```python
from build123d import *

# Parameters (mm, degrees)
SKETCH3_R                 = 2.5
BOSS_EXTRUDE1_DEPTH       = 62.34264779
CHAMFER1_SIZE             = 1.5
CHAMFER1_SIZE2            = 0.866025404
M3X0_5_TAPPED_HOLE1_D     = 2.5
M3X0_5_TAPPED_HOLE1_DEPTH = 4
M3X0_5_TAPPED_HOLE1_TIP   = 0.751075774
SKETCH7_R                 = 1.5
CUT_EXTRUDE1_DEPTH        = 3.5
CUT_EXTRUDE1_DEPTH_BACK   = 3.5
SKETCH8_W                 = 1
SKETCH8_H                 = 6
CUT_EXTRUDE2_DEPTH        = 3.5000001
CUT_EXTRUDE2_DEPTH_BACK   = 3.5000001
SKETCH9_R                 = 3
SKETCH9_R_2               = 2
CUT_EXTRUDE3_DEPTH        = 0.75


with BuildPart() as part:
    # Sketch3 → Boss-Extrude1 (new body)
    with BuildSketch(Plane(origin=(0, 0, 0), x_dir=(1, 0, 0), z_dir=(0, 1, 0))):
        Circle(SKETCH3_R)
    extrude(amount=BOSS_EXTRUDE1_DEPTH)

    # Chamfer1
    chamfer1_edges = [part.edges().sort_by_distance(p)[0] for p in [
        (-2.5, 62.34264779, 0),
    ]]
    chamfer1_side = [part.faces().sort_by_distance(p)[0] for p in [
        (-2.5, 31.171323895, 0),
    ]]
    chamfer(chamfer1_edges, length=CHAMFER1_SIZE, length2=CHAMFER1_SIZE2, reference=chamfer1_side[0])

    # M3x0.5 Tapped Hole1
    with Locations(Plane(origin=(0, 62.34264779, 0), x_dir=(1, 0, 0), z_dir=(0, 1, 0))):
        with Locations((0, 0)):
            Hole(M3X0_5_TAPPED_HOLE1_D / 2, depth=M3X0_5_TAPPED_HOLE1_DEPTH)
            with Locations((0, 0, -(M3X0_5_TAPPED_HOLE1_DEPTH + M3X0_5_TAPPED_HOLE1_TIP / 2))):  # 118° drill point
                Cone(0, M3X0_5_TAPPED_HOLE1_D / 2, M3X0_5_TAPPED_HOLE1_TIP, mode=Mode.SUBTRACT)

    # Sketch7 → Cut-Extrude1 (cut, two sides)
    with BuildSketch(Plane.XY) as cut_extrude1_sk:
        with Locations((0, 58.34264779)):
            Circle(SKETCH7_R)
    extrude(amount=CUT_EXTRUDE1_DEPTH, mode=Mode.SUBTRACT)
    extrude(cut_extrude1_sk.sketch, amount=-CUT_EXTRUDE1_DEPTH_BACK, mode=Mode.SUBTRACT)

    # Sketch8 → Cut-Extrude2 (cut, two sides)
    with BuildSketch(Plane.XY) as cut_extrude2_sk:
        with Locations((-2, 3)):
            Rectangle(SKETCH8_W, SKETCH8_H)
    extrude(amount=CUT_EXTRUDE2_DEPTH, mode=Mode.SUBTRACT)
    extrude(cut_extrude2_sk.sketch, amount=-CUT_EXTRUDE2_DEPTH_BACK, mode=Mode.SUBTRACT)

    # Sketch9 → Cut-Extrude3 (cut)
    with BuildSketch(Plane(origin=(0, 17.15, 0), x_dir=(1, 0, 0), z_dir=(0, 1, 0))):
        Circle(SKETCH9_R)
        Circle(SKETCH9_R_2, mode=Mode.SUBTRACT)
    extrude(amount=CUT_EXTRUDE3_DEPTH, mode=Mode.SUBTRACT)


solid = part.part
```
Can you work these out from the model? Positions are in its coordinate system, mm. A direction names the side the tool comes from. Give positions to 0.01 mm unless a question says otherwise; leave off trailing zeros. Loops run counter-clockwise (first coordinate to the right, second up) from the corner with the lowest first, then second, coordinate; pieces in that order, holes last. Notation, with made-up numbers: M -9.5,-38 L -2.5,-38 A23 cw -2.5,1 Z; hole C 85.25,-26.75 d7. An arc over 180 degrees is marked long. Answer in a Markdown table with one row per item.
1. Thinking about a two-plate mould opening in Y: for faces 5 (the cylindrical face through (2.385, 8.455, -0.751)), 6 (the flat face through (1, 62.343, 1)), 7 (the cylindrical face through (-0.434, 17.52, 1.952)), which applies, released by +Y, released by -Y, zero draft, split by the parting line, or undercut?
Taken from the geometry:
| item | result |
|---|---|
| face 5 | zero draft |
| face 6 | released by +Y |
| face 7 | undercut |
2. Suppose I cut it at B-B on z = 0. Write out the boundary of the cut face in (x, y), plus the area to 3 significant figures.
Taken from the geometry:
| item | result |
|---|---|
| outline | M -2.5,6 L -1.5,6 L -1.5,0 L 2.5,0 L 2.5,17.15 L 2,17.15 L 2,17.9 L 2.5,17.9 L 2.5,60.84 L 1.63,62.34 L 1.25,62.34 L 1.25,59.17 A1.5 cw long -1.25,59.17 L -1.25,62.34 L -1.63,62.34 L -2.5,60.84 L -2.5,17.9 L -2,17.9 L -2,17.15 L -2.5,17.15 Z |
| area | 290 mm² |
3. Suppose I cut it at A-A on x = 0. Write out the boundary of the cut face in (y, z), plus the area to 3 significant figures.
Taken from the geometry:
| item | result |
|---|---|
| outline | M 0,-2.5 L 17.15,-2.5 L 17.15,-2 L 17.9,-2 L 17.9,-2.5 L 56.84,-2.5 L 56.84,2.5 L 17.9,2.5 L 17.9,2 L 17.15,2 L 17.15,2.5 L 0,2.5 Z; M 59.84,-2.5 L 60.84,-2.5 L 62.34,-1.63 L 62.34,-1.25 L 59.84,-1.25 Z; M 59.84,1.25 L 62.34,1.25 L 62.34,1.63 L 60.84,2.5 L 59.84,2.5 Z |
| area | 288 mm² |
4. For pin 1 Ø1 at (y, z) = (21.5, 2) entering from +X; pin 2 Ø3 at (y, z) = (3.5, 0) entering from -X; pin 3 Ø0.8 at (x, z) = (-2, 0) entering from -Y, each with a flat end and sliding along its axis, tell me the tip position at first contact or that it passes through.
Taken from the geometry:
| item | result |
|---|---|
| pin 1 | stops at x = 2 |
| pin 2 | stops at x = -1.5 |
| pin 3 | stops at y = 6 |
5. If I drill on line 1 along Z through (x, y) = (0, 60); line 2 along Y through (x, z) = (0, 0.75); line 3 along Y through (x, z) = (1.2, 2.1), over which ranges is the centre line in solid material (lowest first)?
Taken from the geometry:
| item | result |
|---|---|
| line 1 | z = -2.5 to -1.25, 1.25 to 2.5 |
| line 2 | y = 0 to 56.84 |
| line 3 | y = 0 to 17.15, 17.9 to 57.44, 59.24 to 60.98 |
6. Suppose I cut it at C-C on y = 19. Write out the boundary of the cut face in (x, z), plus the area to 3 significant figures.
Taken from the geometry:
| item | result |
|---|---|
| outline | C 0,0 d5 |
| area | 19.6 mm² |
7. Which directions (+Z, -Z, +X, -X, +Y, -Y) give clear straight access to the entire face, cutting with the end or side of a thin tool? Please do faces 1 (the flat face through (-1.5, 3, 0)), 2 (the flat face through (0, 0, 0)), 3 (the flat face through (-1, 17.15, -2)), 4 (the cylindrical face through (-1.155, 61.087, 0.479)).
Taken from the geometry:
| item | result |
|---|---|
| face 1 | +Z, -Z, -X, -Y |
| face 2 | +Z, -Z, +X, -X, -Y |
| face 3 | none |
| face 4 | +Y |
